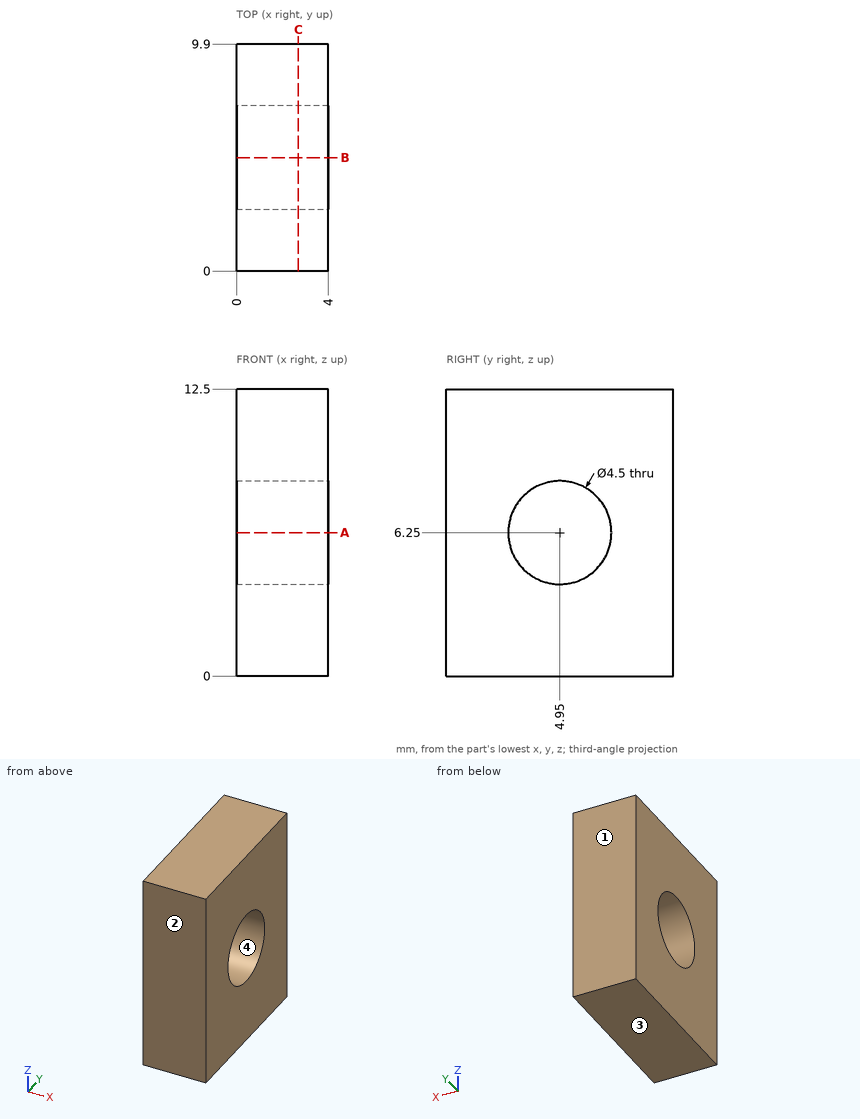
The drawing under review shows one solid part. Ordinate dimensions are in mm from its lowest x, y, z. Round coordinates to 2 decimals unless told otherwise and drop trailing zeros. Loops run counter-clockwise (first coordinate to the right, second up) from the corner with the lowest first, then second, coordinate; pieces in that order, holes last. Notation, with made-up numbers: (18.25, -20) - (53.25, -20) arc R15 cw to (53.25, 5) - close; hole circle Ø2 at (37.25, 51). An arc over 180 degrees is marked (long way). Use one line per item in the form item = value.
Item 1: Consider section B-B on y = 4.95. Write out the cut boundary in (x, z), then the cut area to 3 significant figures.
Answers:
outline = (0, 0) - (4, 0) - (4, 4) - (0, 4) - close; (0, 8.5) - (4, 8.5) - (4, 12.5) - (0, 12.5) - close
area = 32.0 mm^2
Item 2: Consider section C-C on x = 2.7. Write out the cut boundary in (y, z).
Answers:
outline = (0, 0) - (9.9, 0) - (9.9, 12.5) - (0, 12.5) - close; hole circle Ø4.5 at (4.95, 6.25)
Item 3: Consider section A-A on z = 6.25. Write out the cut boundary in (x, y), then the cut area to 3 significant figures.
Answers:
outline = (0, 0) - (4, 0) - (4, 2.7) - (0, 2.7) - close; (0, 7.2) - (4, 7.2) - (4, 9.9) - (0, 9.9) - close
area = 21.6 mm^2
Item 4: For line 1 (Z direction, x = 0.9, y = 5); line 2 (Y direction, x = 1, z = 8.25); line 3 (Y direction, x = 3, z = 6), list the stretches that pass through material, from the lowest coordinate up.
Answers:
line_1 = 0 to 4, 8.5 to 12.5
line_2 = 0 to 3.92, 5.98 to 9.9
line_3 = 0 to 2.71, 7.19 to 9.9
Item 5: Clearance check with a flat-ended pin moving along its axis: P1, Ø3, axis at y = 3, z = 6.5, coming from the +X side. State where the tip first meets the part, or that it passes through.
Answers:
P1 = 4
Item 6: Mouldability with a two-part tool opening along Y and no side actions: class the marked faces 1, 2, 3 and 4 as +Y half, -Y half, draft (parallel to the pull), parting line (faces both ways), or undercut.
Answers:
face_1 = +Y half
face_2 = -Y half
face_3 = draft
face_4 = undercut
